Build history of the part. All positions in model axes, mm. Face numbers are marked on the shaded views. A direction names the side the tool comes from. Give positions to 0.01 mm unless a question says otherwise; leave off trailing zeros. Loops run counter-clockwise (first coordinate to the right, second up) from the corner with the lowest first, then second, coordinate; pieces in that order, holes last. Notation, with made-up numbers: M 71.25,-23.5 L 129.25,-23.5 A17 ccw 129.25,-5.5 Z; hole C -27.75,-12 d7. An arc over 180 degrees is marked long. Put each result on its own line as item: value.
```python
from build123d import *

# Parameters (mm, degrees)
F2_DEPTH      = 20
F2_DEPTH_BACK = 20
F3_START      = -25.4
F3_DEPTH      = 59.436


with BuildPart() as f2:
    # F0 (on Front) → F2 (new body, two sides)
    with BuildSketch(Plane.XZ) as f2_sk:
        with BuildLine():
            Line((0, -4), (20, -4))
            Line((20, -4), (20, 3))
            ThreePointArc((20, 3), (19.7071067812, 3.7071067812), (19, 4))
            Line((19, 4), (17.4655668493, 4))
            ThreePointArc((17.4655668493, 4), (16.7822617025, 4.269867083), (16.4677596893, 4.9338118471))
            Line((16.4677596893, 4.9338118471), (15.0045070864, 26.9928036795))
            ThreePointArc((15.0045070864, 26.9928036795), (10.2733190387, 36.9647668796), (0, 41))
            ThreePointArc((0, 41), (-10.2733190387, 36.9647668796), (-15.0045070864, 26.9928036795))
            Line((-15.0045070864, 26.9928036795), (-16.4677596893, 4.9338118471))
            ThreePointArc((-16.4677596893, 4.9338118471), (-16.7822617025, 4.269867083), (-17.4655668493, 4))
            Line((-17.4655668493, 4), (-19, 4))
            ThreePointArc((-19, 4), (-19.7071067812, 3.7071067812), (-20, 3))
            Line((-20, 3), (-20, -4))
            Line((-20, -4), (0, -4))
        make_face()
        with BuildLine():
            ThreePointArc((10.0373301632, 25.9999767743), (7.0863665619, 18.90694598), (-0.0248870067, 16.000170325))
            ThreePointArc((-0.0248870067, 16.000170325), (-7.0117062355, 33.0930075686), (10.0373301632, 25.9999767743))
        make_face(mode=Mode.SUBTRACT)
    extrude(amount=F2_DEPTH)
    extrude(f2_sk.sketch, amount=-F2_DEPTH_BACK)

    # F1 (on Right) → F3 (intersect)
    with BuildSketch(Plane.YZ.offset(F3_START)):
        with BuildLine():
            ThreePointArc((20, 2), (19.4142135624, 3.4142135624), (18, 4))
            Line((18, 4), (15, 4))
            Line((15, 4), (14, 4))
            Line((14, 4), (10, 4))
            Line((10, 4), (-15, 4))
            Line((-15, 4), (-20, 4))
            Line((-20, 4), (-20, -4))
            Line((-20, -4), (20, -4))
            Line((20, -4), (20, 2))
        make_face()
        Polygon((14, 4), (15, 4), (15, 41), (14.5, 41), (14, 41), (10, 35), (10, 4), align=None)
        with BuildLine():
            Line((-20, 4), (-15, 4))
            Line((-15, 4), (-15, 41))
            ThreePointArc((-15, 41), (-18.5355339059, 39.5355339059), (-20, 36))
            Line((-20, 36), (-20, 4))
        make_face()
    extrude(amount=F3_DEPTH, mode=Mode.INTERSECT)


solid = f2.part
```
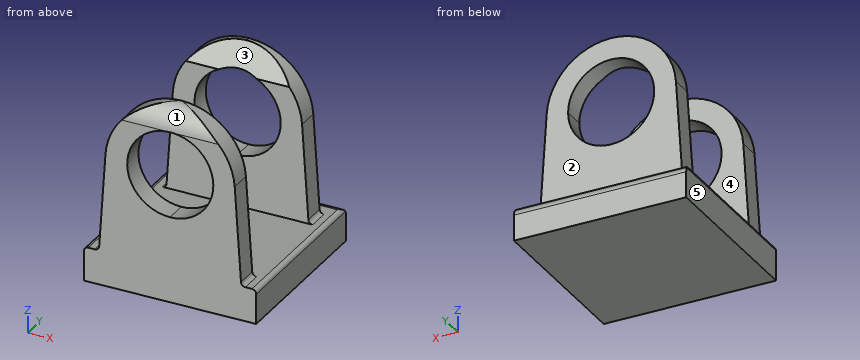
Q1. Slice it at A-A (y = -2.5). List the corners of the cut face in (x, z), and give its area (3 significant figures).
Here are the results:
outline: M -20,-4 L 20,-4 L 20,3 A1 ccw 19,4 L -19,4 A1 ccw -20,3 Z
area: 320 mm²
Q2. Tool access for the marked faces 4 and 5: list every direction of +Z, -Z, +X, -X, +Y, -Y with a clear straight run to the whole face (end or side of a thin tool).
Here are the results:
face 4: +Z, +X, -X
face 5: +Z, -Z, -X, +Y, -Y
Q3. Slice it at D-D (y = 12.5). List the corners of the cut face in (x, z).
Here are the results:
outline: M -20,-4 L 20,-4 L 20,3 A1 ccw 19,4 L 17.47,4 A1 cw 16.47,4.93 L 15,26.99 A15 ccw 7.94,38.75 L -7.94,38.75 A15 ccw -15,26.99 L -16.47,4.93 A1 cw -17.47,4 L -19,4 A1 ccw -20,3 Z; hole C 0.04,26 d20
Q4. Mould opens along Y. For the marked faces 1, 2 and 3 say: pulls with the +Y half, pulls with the -Y half, needs draft (parallel to the pull), parting line crosses it, or undercut.
Here are the results:
face 1: pulls with the -Y half
face 2: pulls with the +Y half
face 3: undercut
Q5. Drop flat-ended pins along their axis: pin 1 Ø12 at (y, z) = (5, 26.5) entering from -X; pin 2 Ø1 at (x, y) = (-14.5, -5) entering from +Z; pin 3 Ø17.5 at (x, z) = (4.5, 24) entering from +Y. Give the stop position or say it passes through.
Here are the results:
pin 1: x = -15.26
pin 2: z = 4
pin 3: y = 15
Q6. Slice it at C-C (x = 5). List the corners of the cut face in (y, z), and give its area (3 significant figures).
Here are the results:
outline: M -20,-4 L 20,-4 L 20,2 A2 ccw 18,4 L 15,4 L 15,17.32 L 10,17.32 L 10,4 L -15,4 L -15,17.32 L -20,17.32 Z; M -20,34.68 L -15,34.68 L -15,40.16 L -17.78,40.16 A5 ccw -20,36 Z; M 10,34.68 L 15,34.68 L 15,40.16 L 13.44,40.16 L 10,35 Z
area: 495 mm²
Q7. Probe line 1 (Y direction, x = 11, z = 22.5); line 2 (Z direction, x = 7, y = 2); line 3 (Z direction, x = -4.5, y = 11). List the from-to ranges inside material, lowest first. Write a range as from..to.
Here are the results:
line 1: -20..-15, 10..15
line 2: -4..4
line 3: -4..17.09, 34.91..36.5
Q8. Slice it at B-B (z = 9). List the corners of the cut face in (x, y), and give its area (3 significant figures).
Here are the results:
outline: M -16.2,-20 L 16.2,-20 L 16.2,-15 L -16.2,-15 Z; M -16.2,10 L 16.2,10 L 16.2,15 L -16.2,15 Z
area: 324 mm²
